Build history of the part. All positions in model axes, mm. A direction names the side the tool comes from. Round coordinates to 2 decimals unless told otherwise and drop trailing zeros. Loops run counter-clockwise (first coordinate to the right, second up) from the corner with the lowest first, then second, coordinate; pieces in that order, holes last. Notation, with made-up numbers: (83, 24.5) -> (130, 24.5) arc R29 ccw to (130, 61.5) -> close; hole circle Ø1 at (47.5, 47). An arc over 180 degrees is marked (long way). Put each result on its own line as item: value. Start each with the question number.
Item 1: Cut at A-A, the plane z = 11.5. List the corners of the cut face in (x, y).
Item 2: Drill centre lines: probe 1 along Y at (x, z) = (42.5, 6.5); probe 2 along Y at (x, z) = (-42.5, 7); probe 3 along Y at (x, z) = (45, 3.25). Where is each one in solid material? Low to high. Write a range as [from, to].
Item 3: Tool access for faces 1 (the flat face through (-44, -25, 8.2)), 2 (the flat face through (52, -5.05, 4)), 3 (the cylindrical face through (-44.405, 23.54, 5.057)): list every direction of +Z, -Z, +X, -X, +Y, -Y with a clear straight run to the whole face (end or side of a thin tool).
Item 4: Flat gauge pins, fed straight in: pin 1 Ø8 at (y, z) = (3.5, 10.5) entering from -X; pin 2 Ø4 at (x, z) = (-14, 9.5) entering from -Y; pin 3 Ø1.1 at (y, z) = (-0.5, 14.5) entering from -X; pin 4 Ø6 at (x, z) = (14, 13.5) entering from -Y. Where does each tip first touch, or does it go through?
Item 5: Cut at D-D, the plane x = -2.5. List the corners of the cut face in (y, z), plus the area to 3 significant figures.
Item 6: Pull direction X, two halves, no side cores. Call faces 4 (the flat face through (-53.5, 24, 3)), 5 (the cylindrical face through (41.98, 22.657, 5.057)), 6 (the flat face through (1, 43.85, 3)): +X half, -X half, draft (parallel to the pull), parting line (faces both ways), or undercut.
Item 7: Cut at C-C, the plane y = 38. List the corners of the cut face in (x, z), plus the area to 3 significant figures.
```python
from build123d import *

# Parameters (mm, degrees)
SKETCH_W      = 102.2
SKETCH_H      = 83
SKETCH_W_2    = 30
SKETCH_H_2    = 5
SKETCH_W_3    = 2
SKETCH_H_3    = 25
PAD_DEPTH     = 2
SKETCH001_R   = 2.4
SKETCH001_R_2 = 1.2
PAD001_DEPTH  = 6.2
PAD002_DEPTH  = 6.9
PAD003_DEPTH  = 1
SKETCH004_W   = 1.45
SKETCH004_H   = 11.2
PAD004_DEPTH  = 5
SKETCH005_W   = 1.45
SKETCH005_H   = 5
PAD005_DEPTH  = 7
PAD006_DEPTH  = 5
FILLET_R      = 1
FILLET001_R   = 1
FILLET002_R   = 1
FILLET003_R   = 1


with BuildPart() as part:
    # Sketch → Pad (new body)
    with BuildSketch(Plane.XY):
        Rectangle(SKETCH_W, SKETCH_H)
        with Locations((34.1, 17.5)):
            Rectangle(SKETCH_W_2, SKETCH_H_2, mode=Mode.SUBTRACT)
        with Locations((-34.1, 17.5)):
            Rectangle(SKETCH_W_2, SKETCH_H_2, mode=Mode.SUBTRACT)
        with Locations((6, -27)):
            Rectangle(SKETCH_W_3, SKETCH_H_3, mode=Mode.SUBTRACT)
        with Locations((-6, -27)):
            Rectangle(SKETCH_W_3, SKETCH_H_3, mode=Mode.SUBTRACT)
    extrude(amount=PAD_DEPTH)

    # Sketch001 (on Face22 of Pad) → Pad001 (join)
    with BuildSketch(Plane.XY.offset(2)):
        with Locations((-42.5, -25)):
            Circle(SKETCH001_R)
        with Locations((-42.5, -25)):
            Circle(SKETCH001_R_2, mode=Mode.SUBTRACT)
        with Locations((42.5, 25)):
            Circle(SKETCH001_R)
        with Locations((42.5, 25)):
            Circle(SKETCH001_R_2, mode=Mode.SUBTRACT)
        with Locations((42.25, -25)):
            Circle(SKETCH001_R)
        with Locations((42.25, -25)):
            Circle(SKETCH001_R_2, mode=Mode.SUBTRACT)
        with Locations((-42.5, 25)):
            Circle(SKETCH001_R)
        with Locations((-42.5, 25)):
            Circle(SKETCH001_R_2, mode=Mode.SUBTRACT)
    extrude(amount=PAD001_DEPTH)

    # Sketch002 → Pad002 (join)
    with BuildSketch(Plane.XY):
        Polygon((-51.1, 41.5), (51.1, 41.5), (51.1, 5.05), (53.5, 5.05), (53.5, 43.85), (-53.5, 43.85), (-53.5, 5.05), (-51.1, 5.05), align=None)
    pad002 = extrude(amount=PAD002_DEPTH)

    # Mirrored: Pad002 across XZ
    add(pad002.mirror(Plane.XZ))

    # Sketch003 (on Face38 of Mirrored) → Pad003 (join)
    with BuildSketch(Plane.XY.offset(6.9)):
        Polygon((-51.1, 5.05), (-51.1, 41.5), (51.1, 41.5), (51.1, 5.05), (52.1, 5.05), (52.1, 42.5), (-52.1, 42.5), (-52.1, 5.05), align=None)
    pad003 = extrude(amount=PAD003_DEPTH)

    # Mirrored001: Pad003 across XZ
    add(pad003.mirror(Plane.XZ))

    # Sketch004 (on Face3 of Mirrored001) → Pad004 (join)
    with BuildSketch(Plane.XY.offset(2)):
        with Locations((50.375, 0)):
            Rectangle(SKETCH004_W, SKETCH004_H)
    pad004 = extrude(amount=PAD004_DEPTH)

    # Mirrored002: Pad004 across YZ
    add(pad004.mirror(Plane.YZ))

    # Sketch005 (on Face40 of Mirrored002) → Pad005 (join)
    with BuildSketch(Plane.XY.offset(7)):
        with Locations((50.375, 0)):
            Rectangle(SKETCH005_W, SKETCH005_H)
    pad005 = extrude(amount=PAD005_DEPTH)

    # Mirrored003: Pad005 across YZ
    add(pad005.mirror(Plane.YZ))

    # Sketch006 (on Face2 of Mirrored003) → Pad006 (join)
    with BuildSketch(Plane.XZ.offset(2.5)):
        Polygon((49.65, 14), (51.1, 14), (53.1, 14), (53.1, 15), (51.15, 18), (49.65, 18), align=None)
    pad006 = extrude(amount=-PAD006_DEPTH)

    # Mirrored004: Pad006 across YZ
    add(pad006.mirror(Plane.YZ))

    # Fillet
    fillet_edges = [part.edges().sort_by_distance(p)[0] for p in [
        (53.5, -43.85, 3.45),
    ]]
    fillet(fillet_edges, radius=FILLET_R)

    # Fillet001
    fillet001_edges = [part.edges().sort_by_distance(p)[0] for p in [
        (53.5, 43.85, 3.45),
    ]]
    fillet(fillet001_edges, radius=FILLET001_R)

    # Fillet002
    fillet002_edges = [part.edges().sort_by_distance(p)[0] for p in [
        (-53.5, -43.85, 3.45),
    ]]
    fillet(fillet002_edges, radius=FILLET002_R)

    # Fillet003
    fillet003_edges = [part.edges().sort_by_distance(p)[0] for p in [
        (-53.5, 43.85, 3.45),
    ]]
    fillet(fillet003_edges, radius=FILLET003_R)


solid = part.part
```
Reply:
1. outline: (-51.1, -2.5) -> (-49.65, -2.5) -> (-49.65, 2.5) -> (-51.1, 2.5) -> close; (49.65, -2.5) -> (51.1, -2.5) -> (51.1, 2.5) -> (49.65, 2.5) -> close
2. probe 1: y = [-43.85, -41.5], [-27.39, -26.17], [-23.83, -22.61], [22.6, 23.8], [26.2, 27.4], [41.5, 43.85]
2. probe 2: y = [-42.5, -41.5], [-27.4, -26.2], [-23.8, -22.6], [22.6, 23.8], [26.2, 27.4], [41.5, 42.5]
2. probe 3: y = [-43.85, -41.5], [41.5, 43.85]
3. face 1: +Z, +X, -X, +Y, -Y
3. face 2: +Z, -Z, +X
3. face 3: +Z
4. pin 1: stops at x = -53.5
4. pin 2: stops at y = -42.5
4. pin 3: stops at x = -53.1
4. pin 4: passes through
5. outline: (-43.85, 0) -> (43.85, 0) -> (43.85, 6.9) -> (42.5, 6.9) -> (42.5, 7.9) -> (41.5, 7.9) -> (41.5, 2) -> (-41.5, 2) -> (-41.5, 7.9) -> (-42.5, 7.9) -> (-42.5, 6.9) -> (-43.85, 6.9) -> close
5. area: 200 mm^2
6. face 4: -X half
6. face 5: undercut
6. face 6: draft
7. outline: (-53.5, 0) -> (53.5, 0) -> (53.5, 6.9) -> (52.1, 6.9) -> (52.1, 7.9) -> (51.1, 7.9) -> (51.1, 2) -> (-51.1, 2) -> (-51.1, 7.9) -> (-52.1, 7.9) -> (-52.1, 6.9) -> (-53.5, 6.9) -> close
7. area: 240 mm^2
